Study the drawing (mm; zero at the part's minimum x, y, z) and answer. A direction names the side the tool comes from. Coordinates: 2 decimals unless noted, no trailing zeros. Loops run counter-clockwise (first coordinate to the right, second up) from the corner with the lowest first, then second, coordinate; pieces in that order, holes last. Notation, with made-up numbers: (-20.5, -7.5) -> (-15.5, -7.5) arc R27 ccw to (-15.5, 11.5) -> close; hole circle Ø3 at (71.25, 72). An arc over 180 degrees is marked (long way). Answer as a JSON object with one key per item and string values. Group by question number.
Q1. The part is cut by section B-B on y = 15.25. Write down the section's boundary in (x, z).
Q2. For the marked faces 3, 4 and 5, determine the directions among +Z, -Z, +X, -X, +Y, -Y from which every point of the face is accessible in a straight line to the end or side of a thin tool.
Q3. Determine the mould class of the marked faces 1 and 2 for opening direction X: released by +X, released by -X, zero draft, split by the parting line, or undercut.
Q4. Straight lines are drawn through the part: line 1 along Y through (x, z) = (22, 0.6); line 2 along Y through (x, z) = (21.5, 3.1); line 3 along X through (y, z) = (6, 0.9). For each, find the intervals that lie inside material, in ascending order. Write a range as [from, to].
Q5. The part is cut by section C-C on x = 4.5. Write down the section's boundary in (y, z).
Q6. The part is cut by section D-D on y = 18.5. Write down the section's boundary in (x, z), and give its area (3 significant figures).
Q7. Each of these flat-tipped pins is pushed along its axis until it touches: P1, Ø3, axis at x = 15, y = 15, coming from the +Z side; P2, Ø1.5, axis at y = 6.5, z = 0.5, coming from the +X side; P3, Ø2.5, axis at x = 4.5, z = 5, coming from the -Y side; P4, Ø2, axis at x = 22.45, y = 6.55, coming from the +Z side. Where does it stop, or does it pass through?
Q8. The part is cut by section A-A on x = 14.5. Write down the section's boundary in (y, z).
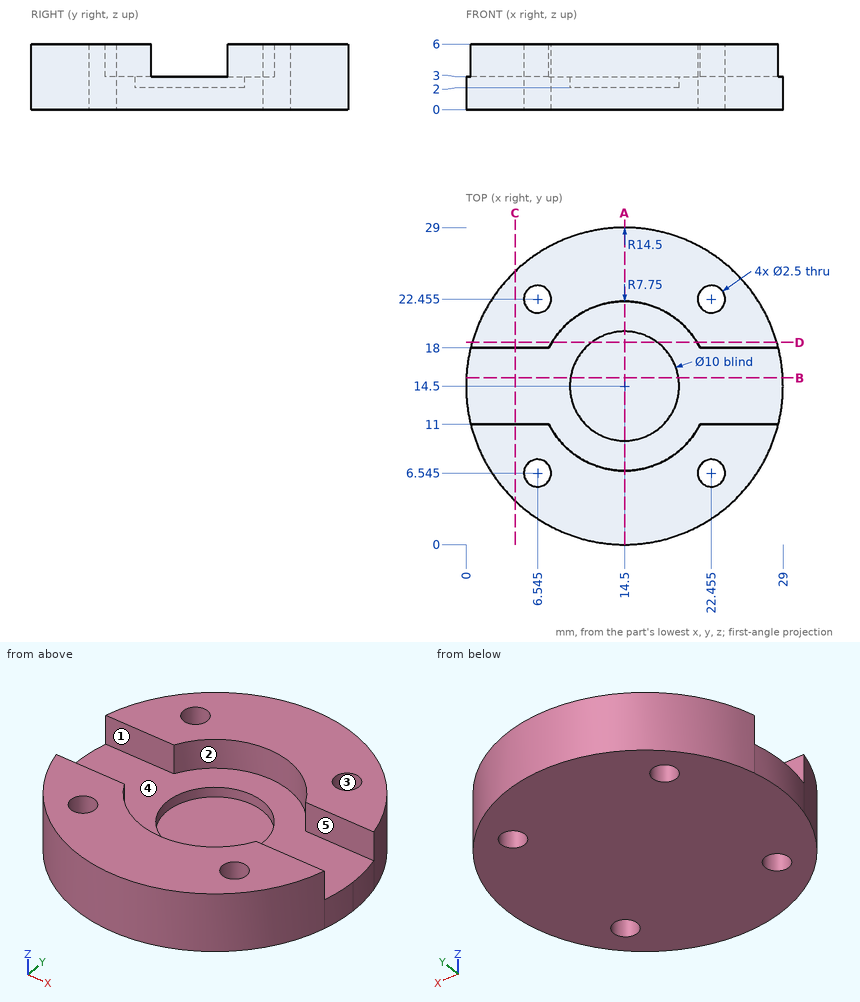
Final values:
{
 "1": {"outline": "(0.02, 0) -> (28.98, 0) -> (28.98, 3) -> (19.44, 3) -> (19.44, 2) -> (9.56, 2) -> (9.56, 3) -> (0.02, 3) -> close"},
 "2": {"face 3": "+Z, -Z", "face 4": "+Z", "face 5": "+Z, +X, -X"},
 "3": {"face 1": "zero draft", "face 2": "undercut"},
 "4": {"line 1": "y = [2.09, 5.38], [7.71, 21.29], [23.62, 26.91]", "line 2": "y = [1.8, 5.74], [7.35, 11], [18, 21.65], [23.26, 27.2]", "line 3": "x = [2.75, 5.42], [7.67, 21.33], [23.58, 26.25]"},
 "5": {"outline": "(4, 0) -> (25, 0) -> (25, 6) -> (18, 6) -> (18, 3) -> (11, 3) -> (11, 6) -> (4, 6) -> close"},
 "6": {"outline": "(0.56, 0) -> (28.44, 0) -> (28.44, 6) -> (21.14, 6) -> (21.14, 3) -> (17.5, 3) -> (17.5, 2) -> (11.5, 2) -> (11.5, 3) -> (7.86, 3) -> (7.86, 6) -> (0.56, 6) -> close", "area": "121 mm2"},
 "7": {"P1": "stops at z = 2", "P2": "stops at x = 27.06", "P3": "stops at y = 2.94", "P4": "passes through"},
 "8": {"outline": "(0, 0) -> (29, 0) -> (29, 6) -> (22.25, 6) -> (22.25, 3) -> (19.5, 3) -> (19.5, 2) -> (9.5, 2) -> (9.5, 3) -> (6.75, 3) -> (6.75, 6) -> (0, 6) -> close"}
}
